```python
from build123d import *

# Parameters (mm, degrees)
F0_W      = 32
F0_H      = 30
F1_DEPTH  = 1.4
F2_W      = 9
F2_H      = 11
F3_DEPTH  = 11
F4_R      = 4.49999
F6_W      = 7
F6_H      = 7
F7_DEPTH  = 6.3
F8_W      = 3.8
F8_H      = 3.8
F9_DEPTH  = 5
F5_W      = 9
F5_H      = 11
F10_DEPTH = 3


# Not quite as in the source:
# - a fillet or chamfer is up to 0.001 mm smaller than in the source, because OpenCascade refuses the exact size


with BuildPart() as f1:
    # F0 (on Front) → F1 (new body)
    with BuildSketch(Plane.XZ):
        Rectangle(F0_W, F0_H)
    extrude(amount=F1_DEPTH)

    # F2 (on face) → F3 (join)
    with BuildSketch(Plane.XZ.offset(1.4)):
        with Locations((-8.9, 9.5)):
            Rectangle(F2_W, F2_H)
    extrude(amount=F3_DEPTH)

    # F4 (radius 4.5 in the source; OpenCascade refuses exactly that, so slightly less here)
    f4_edges = [f1.edges().sort_by_distance(p)[0] for p in [
        (-4.4, -12.4, 9.5),
        (-13.4, -12.4, 9.5),
    ]]
    fillet(f4_edges, radius=F4_R)

    # F6 (on face) → F7 (join)
    with BuildSketch(Plane.XZ.offset(1.4)):
        with Locations((1.7, 7.8)):
            Rectangle(F6_W, F6_H)
    extrude(amount=F7_DEPTH)

    # F8 (on face) → F9 (join)
    with BuildSketch(Plane.XZ.offset(7.7)):
        with Locations((1.7, 7.8)):
            Rectangle(F8_W, F8_H)
    extrude(amount=F9_DEPTH)

    # F5 (on face) → F10 (join)
    with BuildSketch(Plane.XY.offset(15)):
        with Locations((-8.9, -6.9)):
            Rectangle(F5_W, F5_H)
    extrude(amount=F10_DEPTH)


solid = f1.part
```
The model under review builds one solid part; all positions refer to its coordinate system, in mm. A direction names the side the tool comes from. Round coordinates to 2 decimals unless told otherwise and drop trailing zeros. Loops run counter-clockwise (first coordinate to the right, second up) from the corner with the lowest first, then second, coordinate; pieces in that order, holes last. Notation, with made-up numbers: (76, 60) - (130, 60) arc R15 ccw to (130, 86) - close; hole circle Ø9 at (-31, 15). An arc over 180 degrees is marked (long way). Write each question's results on one line, items separated by ' | '. Start each with the question number.
Q1. Insertion check: P1, Ø3.5, axis at x = -6, y = -11, coming from the -Z side; P2, Ø4, axis at y = -7.5, z = 10.5, coming from the +X side; P3, Ø8, axis at x = 8, z = 3, coming from the -Y side. Each pin has a flat end and moves straight along its axis. Give the tip position at first contact, or say it passes through.
Q2. Take a section at D-D on y = -4.25. Give the boundary of the cut face in (x, z).
Q3. Draft analysis for pull direction X (two halves, no side actions). For faces 1 (the cylindrical face through (-5.683, -11.047, 9.577)), 2 (the flat face through (-16, -1, 0)), 3 (the flat face through (2, -12.7, 8)), state which applies: pulls with the +X half, pulls with the -X half, needs draft (parallel to the pull), parting line crosses it, or undercut.
Q4. Tool access review of faces 4 (the flat face through (-9, -7, 4)), 5 (the flat face through (2, -5, 11.3)), 6 (the flat face through (5.2, -5, 8)), 7 (the flat face through (2, -10, 5.9)), 8 (the flat face through (-1.8, -5, 8)): name each direction out of +Z, -Z, +X, -X, +Y, -Y from which nothing blocks a thin tool from reaching the whole face with its end or side.
Q5. Wall thickness on line 1 along Z through (x, y) = (2.5, -1); line 2 along Z through (x, y) = (0, -3); line 3 along Y through (x, z) = (-8, -2): over which ranges is each line inside the solid? List them lowest first. Write a range as [from, to].
Q6. Take a section at A-A on y = -11.5. Give the boundary of the cut face in (x, z).
Q7. Take a section at B-B on x = 3. Give the boundary of the cut face in (y, z), plus the area to 3 significant figures.
Data:
1) P1: stops at z = 4 | P2: stops at x = 5.2 | P3: stops at y = -7.7
2) outline: (-13.4, 4) - (-4.4, 4) - (-4.4, 18) - (-13.4, 18) - close; (-1.8, 4.3) - (5.2, 4.3) - (5.2, 11.3) - (-1.8, 11.3) - close
3) face 1: undercut | face 2: pulls with the -X half | face 3: needs draft
4) face 4: -Z, +X, -X, -Y | face 5: +Z, +X, -Y | face 6: +Z, -Z, +X, -Y | face 7: -Z, +X, -Y | face 8: +Z, -Z, -Y
5) line 1: z = [-15, 15] | line 2: z = [4.3, 11.3] | line 3: y = [-1.4, 0]
6) outline: (-13.4, 15) - (-11.6, 15) - (-11.6, 4) - (-6.2, 4) - (-6.2, 15) - (-4.4, 15) - (-4.4, 18) - (-13.4, 18) - close; (-0.2, 5.9) - (3.6, 5.9) - (3.6, 9.7) - (-0.2, 9.7) - close
7) outline: (-12.7, 5.9) - (-7.7, 5.9) - (-7.7, 4.3) - (-1.4, 4.3) - (-1.4, -15) - (0, -15) - (0, 15) - (-1.4, 15) - (-1.4, 11.3) - (-7.7, 11.3) - (-7.7, 9.7) - (-12.7, 9.7) - close | area: 105 mm²
